```python
from build123d import *

# Parameters (mm, degrees)
SKETCH1_W           = 51
SKETCH1_H           = 23
BOSS_EXTRUDE1_DEPTH = 1
BOSS_EXTRUDE2_DEPTH = 2
SKETCH3_W           = 26
SKETCH3_H           = 7
BOSS_EXTRUDE3_DEPTH = 1.5
SKETCH4_W           = 4.5
SKETCH4_H           = 4.5
CUT_EXTRUDE1_DEPTH  = 2.3


with BuildPart() as part:
    # Sketch1 → Boss-Extrude1 (new body)
    with BuildSketch(Plane.XY):
        with Locations((-25.5, 11.5)):
            Rectangle(SKETCH1_W, SKETCH1_H)
    extrude(amount=BOSS_EXTRUDE1_DEPTH)

    # Sketch2 → Boss-Extrude2 (add)
    with BuildSketch(Plane.XY.offset(1)):
        Polygon((-51, 23), (0, 23), (0, 21.2), (-49.2, 21.2), (-49.2, 1.8), (0, 1.8), (0, 0), (-51, 0), (-51, 1.8), (-51, 21.2), align=None)
    extrude(amount=BOSS_EXTRUDE2_DEPTH)

    # Sketch3 → Boss-Extrude3 (add)
    with BuildSketch(Plane.XY.offset(1)):
        with Locations((-19.5, 14.5)):
            Rectangle(SKETCH3_W, SKETCH3_H)
    extrude(amount=BOSS_EXTRUDE3_DEPTH)

    # Sketch4 → Cut-Extrude1 (cut)
    with BuildSketch(Plane.XY.offset(2.5)):
        with Locations((-29, 14.5)):
            Rectangle(SKETCH4_W, SKETCH4_H)
        with Locations((-22.666666667, 14.5)):
            Rectangle(SKETCH4_W, SKETCH4_H)
        with Locations((-16.333333333, 14.5)):
            Rectangle(SKETCH4_W, SKETCH4_H)
        with Locations((-10, 14.5)):
            Rectangle(SKETCH4_W, SKETCH4_H)
    extrude(amount=-CUT_EXTRUDE1_DEPTH, mode=Mode.SUBTRACT)


solid = part.part
```
For this review, take the finished solid that the model builds, in its own axes (mm). A direction names the side the tool comes from. Give positions to 0.01 mm unless a question says otherwise; leave off trailing zeros. Write each loop counter-clockwise with the first axis right and the second up, starting at its lowest first coordinate (ties: lowest second). Pieces come first, ordered by that corner, then holes. Notation, with made-up numbers: M 34.25,55 L 88.25,55 A16 cw 88.25,81 Z; hole C 79.25,-10 d10. An arc over 180 degrees is marked long. One line per item, written item: value.
1) For line 1 (X direction, y = 14.75, z = 1.05); line 2 (X direction, y = 12.5, z = 0.35); line 3 (Y direction, x = -22, z = 1.95), list the stretches that pass through material, from the lowest coordinate up. Write a range as from..to.
Results are:
line 1: x = -51..-49.2, -32.5..-31.25, -26.75..-24.92, -20.42..-18.58, -14.08..-12.25, -7.75..-6.5
line 2: x = -51..-31.25, -26.75..-24.92, -20.42..-18.58, -14.08..-12.25, -7.75..0
line 3: y = 0..1.8, 11..12.25, 16.75..18, 21.2..23
2) Take a section at D-D, the plane x = -26. Write out the cut boundary in (y, z), then the cut area to 3 significant figures.
Results are:
outline: M 0,0 L 23,0 L 23,3 L 21.2,3 L 21.2,1 L 18,1 L 18,2.5 L 11,2.5 L 11,1 L 1.8,1 L 1.8,3 L 0,3 Z
area: 40.7 mm²
3) Take a section at B-B, the plane x = -4. Write out the cut boundary in (y, z).
Results are:
outline: M 0,0 L 23,0 L 23,3 L 21.2,3 L 21.2,1 L 1.8,1 L 1.8,3 L 0,3 Z
4) The part is to be moulded in two halves that separate along Y. For faces 1 (the flat face through (-23, 15, 0.2)), 2 (the flat face through (0, 11.7, 0.8)), 3 (the flat face through (-25, 0, 1)), 4 (the flat face through (-20, 11, 2)), say which applies: +Y half, -Y half, draft (parallel to the pull), parting line (faces both ways), or undercut.
Results are:
face 1: undercut
face 2: draft
face 3: -Y half
face 4: undercut
5) For faces 5 (the flat face through (-51, 12, 1)), 6 (the flat face through (-24.917, 14, 1)), 7 (the flat face through (-20, 18, 2)), list the 3-axis set-ups (+Z, -Z, +X, -X, +Y, -Y) from which the entire face can be reached by the end or side of a thin tool; tool diameter is ignored.
Results are:
face 5: +Z, -Z, -X, +Y, -Y
face 6: +Z
face 7: +Z, +X
6) Take a section at A-A, the plane z = 1.45. Write out the cut boundary in (x, y), then the cut area to 3 significant figures.
Results are:
outline: M -51,0 L 0,0 L 0,1.8 L -49.2,1.8 L -49.2,21.2 L 0,21.2 L 0,23 L -51,23 Z; M -32.5,11 L -6.5,11 L -6.5,18 L -32.5,18 Z; hole M -31.25,12.25 L -26.75,12.25 L -26.75,16.75 L -31.25,16.75 Z; hole M -24.92,12.25 L -20.42,12.25 L -20.42,16.75 L -24.92,16.75 Z; hole M -18.58,12.25 L -14.08,12.25 L -14.08,16.75 L -18.58,16.75 Z; hole M -12.25,12.25 L -7.75,12.25 L -7.75,16.75 L -12.25,16.75 Z
area: 320 mm²
7) For P1, Ø1, axis at y = 15, z = 2, coming from the +X side; P2, Ø12, axis at x = -42.5, y = 12.5, coming from the +Z side; P3, Ø2, axis at x = -15.5, y = 14.5, coming from the +Z side, all flat-tipped, find the tip position at first contact; note any pin that passes through.
Results are:
P1: stops at x = -6.5
P2: stops at z = 1
P3: stops at z = 0.2
8) Take a section at C-C, the plane y = 2.5. Write out the cut boundary in (x, z), then the cut area to 3 significant figures.
Results are:
outline: M -51,0 L 0,0 L 0,1 L -49.2,1 L -49.2,3 L -51,3 Z
area: 54.6 mm²
